from build123d import *

# Parameters (mm, degrees)
F0_W     = 80
F0_H     = 30
F1_DEPTH = 5
F2_W     = 7.5
F2_H     = 10
F3_DEPTH = 25
F4_W     = 27.5
F4_H     = 10
F5_DEPTH = 5
F6_SIZE  = 14.99999
F7_R     = 5


# Not quite as in the source:
# - a fillet or chamfer is up to 0.001 mm smaller than in the source, because OpenCascade refuses the exact size


with BuildPart() as f1:
    # F0 (on Top) → F1 (new body)
    with BuildSketch(Plane.XY):
        with Locations((3.5, 0)):
            Rectangle(F0_W, F0_H)
    extrude(amount=F1_DEPTH)

    # F2 (on face) → F3 (cut)
    with BuildSketch(Plane.XY.offset(5)):
        with Locations((-10.75, 0)):
            Rectangle(F2_W, F2_H)
    extrude(amount=-F3_DEPTH, mode=Mode.SUBTRACT)

    # F4 (on face) → F5 (cut)
    with BuildSketch(Plane.XY.offset(5)):
        with Locations((25.75, 0)):
            Rectangle(F4_W, F4_H)
    extrude(amount=-F5_DEPTH, mode=Mode.SUBTRACT)

    # F6 (size 15 in the source; OpenCascade refuses exactly that, so slightly less here)
    f6_edges = [f1.edges().sort_by_distance(p)[0] for p in [
        (-36.5, -15, 2.5),
        (-36.5, 15, 2.5),
    ]]
    chamfer(f6_edges, length=F6_SIZE)

    # F7
    f7_edges = [f1.edges().sort_by_distance(p)[0] for p in [
        (43.5, -15, 2.5),
        (43.5, 15, 2.5),
    ]]
    fillet(f7_edges, radius=F7_R)


solid = f1.part
Work out the finished part from the listing and answer in its coordinate system (mm). A direction names the side the tool comes from. Give positions to 0.01 mm unless a question says otherwise; leave off trailing zeros. Write each loop counter-clockwise with the first axis right and the second up, starting at its lowest first coordinate (ties: lowest second). Pieces come first, ordered by that corner, then holes.
Q1. The part is cut by section B-B on x = 17. Give the vertices of the cut face in (y, z), and give its area (3 significant figures).
Answer:
outline: (-15, 0) - (-5, 0) - (-5, 5) - (-15, 5) - close; (5, 0) - (15, 0) - (15, 5) - (5, 5) - close
area: 100 mm2
Q2. The part is cut by section C-C on y = 2. Give the vertices of the cut face in (x, z).
Answer:
outline: (-34.5, 0) - (-14.5, 0) - (-14.5, 5) - (-34.5, 5) - close; (-7, 0) - (12, 0) - (12, 5) - (-7, 5) - close; (39.5, 0) - (43.5, 0) - (43.5, 5) - (39.5, 5) - close
Q3. The part is cut by section A-A on z = 2. State how many separate pieces and enclosed holes the cut face has, and give its area (3 significant figures).
Answer:
separate pieces: 1
enclosed holes: 2
area: 1,810 mm2
Q4. A tool of negligible diameter and unlimited length cuts with its end or side. For faces 4 (the face through (8, 15, 2)), 5 (the face through (26, -5, 3)), from which of +Z, -Z, +X, -X, +Y, -Y can it reach the whole face along a straight path? Write none if from no direction.
Answer:
face 4: +Z, -Z, +X, -X, +Y
face 5: +Z, -Z
Q5. Straight lines are drawn through the part: L1, parallel to Y at x = -7.5, z = 4.7; L2, parallel to X at y = -4.5, z = 3.55; L3, parallel to X at y = -2, z = 3.8. For each, find the intervals that lie inside material, in ascending order.
Answer:
L1: y = -15 to -5, 5 to 15
L2: x = -32 to -14.5, -7 to 12, 39.5 to 43.5
L3: x = -34.5 to -14.5, -7 to 12, 39.5 to 43.5
Q6. The part is cut by section D-D on x = -29. Give the vertices of the cut face in (y, z), and give its area (3 significant figures).
Answer:
outline: (-7.5, 0) - (7.5, 0) - (7.5, 5) - (-7.5, 5) - close
area: 75.0 mm2
Q7. For a pull along X with two mould halves and no side action, classify faces 1 (the face through (-14.5, 0, 3)), 2 (the face through (3, 0, 0)), 3 (the face through (43.5, 0, 2)) as released by +X, released by -X, zero draft, split by the parting line, or undercut.
Answer:
face 1: undercut
face 2: zero draft
face 3: released by +X
Q8. Given pin 1 (1.5 mm diameter, centred on y = 1, z = 3, fed in from -X); pin 2 (5 mm diameter, centred on x = -11, y = 2, fed in from +Z), each flat-ended and moving along its own axis, determine where each tip first touches the part or whether it passes through.
Answer:
pin 1: stops at x = -36.25
pin 2: passes through
